Could you check a few things on this model? Use its own coordinates, in mm. Face numbers are marked on the shaded views. A direction names the side the tool comes from. Give positions to 0.01 mm unless a question says otherwise; leave off trailing zeros. Order: outer loops, then holes, each group sorted by start corner. A loop starts at its lowest first (then second) coordinate and runs counter-clockwise, first axis right, second up. Notation, with made-up numbers: (33.25, 73) - (77.25, 73) arc R11 cw to (77.25, 87) - close; hole circle Ø10 at (28, 86). An arc over 180 degrees is marked (long way). Put each result on its own line as item: value.
from build123d import *

# Parameters (mm, degrees)
SKETCH1_R                            = 4.7625
BOSS_EXTRUDE1_DEPTH                  = 25.4
F_10_32_TAPPED_HOLE1_D               = 4.0386
F_10_32_TAPPED_HOLE1_DEPTH           = 11.938
F_10_32_TAPPED_HOLE1_TIP             = 1.213317848
F_10_32_TAPPED_HOLE1_ON_FACE_2_D     = 4.0386
F_10_32_TAPPED_HOLE1_ON_FACE_2_DEPTH = 11.938
F_10_32_TAPPED_HOLE1_ON_FACE_2_TIP   = 1.213317848


with BuildPart() as part:
    # Sketch1 → Boss-Extrude1 (new, symmetric)
    with BuildSketch(Plane(origin=(0, 0, 0), x_dir=(1, 0, 0), z_dir=(0, 1, 0))):
        with Locations(Location((0, 0, 0), (0, 0, 270))):
            Circle(SKETCH1_R)
    extrude(amount=BOSS_EXTRUDE1_DEPTH, both=True)

    # #10-32 Tapped Hole1
    with Locations(Plane(origin=(0, -25.4, 0), x_dir=(0, 0, -1), z_dir=(0, -1, 0))):
        with Locations((0, 0)):
            Hole(F_10_32_TAPPED_HOLE1_D / 2, depth=F_10_32_TAPPED_HOLE1_DEPTH)
            with Locations((0, 0, -(F_10_32_TAPPED_HOLE1_DEPTH + F_10_32_TAPPED_HOLE1_TIP / 2))):  # 118° drill point
                Cone(0, F_10_32_TAPPED_HOLE1_D / 2, F_10_32_TAPPED_HOLE1_TIP, mode=Mode.SUBTRACT)

    # #10-32 Tapped Hole1 on face 2
    with Locations(Plane.ZX.offset(25.4)):
        with Locations((0, 0)):
            Hole(F_10_32_TAPPED_HOLE1_ON_FACE_2_D / 2, depth=F_10_32_TAPPED_HOLE1_ON_FACE_2_DEPTH)
            with Locations((0, 0, -(F_10_32_TAPPED_HOLE1_ON_FACE_2_DEPTH + F_10_32_TAPPED_HOLE1_ON_FACE_2_TIP / 2))):  # 118° drill point
                Cone(0, F_10_32_TAPPED_HOLE1_ON_FACE_2_D / 2, F_10_32_TAPPED_HOLE1_ON_FACE_2_TIP, mode=Mode.SUBTRACT)


solid = part.part
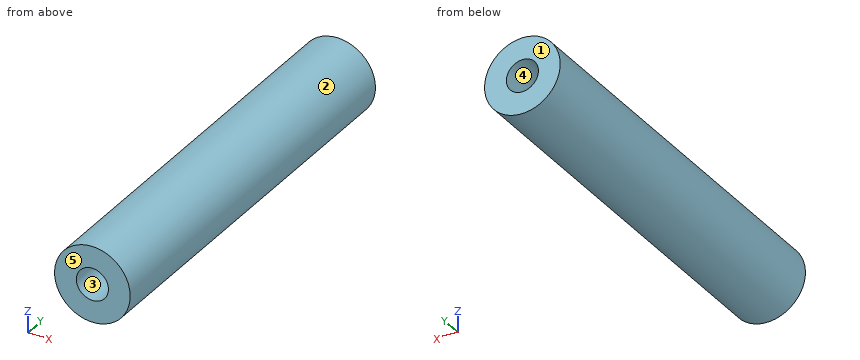
1) Suppose I cut it at D-D, the plane x = -3.5. List the corners of the cut face in (y, z) for me.
Filled in:
outline: (-25.4, -3.23) - (25.4, -3.23) - (25.4, 3.23) - (-25.4, 3.23) - close
2) We'd pull the mould along X, two halves only. Please class the marked faces 1, 2 and 3: pulls with the +X half, pulls with the -X half, needs draft (parallel to the pull), parting line crosses it, or undercut.
Filled in:
face 1: needs draft
face 2: parting line crosses it
face 3: undercut
3) Suppose I cut it at B-B, the plane y = 4.5. List the corners of the cut face in (x, z) for me (1 decimal).
Filled in:
outline: circle Ø9.5 at (0, 0)
4) Suppose I cut it at C-C, the plane z = 3.25. List the corners of the cut face in (x, y) for me.
Filled in:
outline: (-3.48, -25.4) - (3.48, -25.4) - (3.48, 25.4) - (-3.48, 25.4) - close
5) Which directions (+Z, -Z, +X, -X, +Y, -Y) give clear straight access to the entire face, cutting with the end or side of a thin tool? Please do the marked faces 4 and 5.
Filled in:
face 4: +Y
face 5: +Z, -Z, +X, -X, -Y
6) Suppose I cut it at A-A, the plane y = -16. List the corners of the cut face in (x, z) for me (1 decimal), and give its area (3 significant figures).
Filled in:
outline: circle Ø9.5 at (0, 0); hole circle Ø4 at (0, 0)
area: 58.4 mm^2
7) I'm going to push flat-ended pins straight in: pin 1 (2.5 mm diameter, centred on x = 0, z = 0, fed in from -Y); pin 2 (1 mm diameter, centred on x = 3.5, y = -4.5, fed in from +Z); pin 3 (5 mm diameter, centred on y = -17, z = -3, fed in from +X). Where does each tip first touch, or does it pass through?
Filled in:
pin 1: stops at y = -13
pin 2: stops at z = 3.7
pin 3: stops at x = 4.74
8) If I drill on line 1 (X direction, y = 22.25, z = 0); line 2 (X direction, y = -18, z = -0.5); line 3 (X direction, y = 0.5, z = 0.25), over which ranges is the centre line in solid material (lowest first)? Write a range as [from, to].
Filled in:
line 1: x = [-4.76, -2.02], [2.02, 4.76]
line 2: x = [-4.74, -1.96], [1.96, 4.74]
line 3: x = [-4.76, 4.76]
